```python
from build123d import *

# Parameters (mm, degrees)
SKETCH1_R         = 3.8608
EXTRUDE1_DEPTH    = 14.605
SKETCH2_OUTSIDE_W = 13.37
SKETCH2_OUTSIDE_H = 13.37
SKETCH2_OUTSIDE_R = 2.4892
EXTRUDE2_DEPTH    = 9.525
EXTRUDE3_DEPTH    = 3.048


with BuildPart() as part:
    # Sketch1 → Extrude1 (new body)
    with BuildSketch(Plane.XY):
        Circle(SKETCH1_R)
    extrude(amount=EXTRUDE1_DEPTH)

    # Sketch2 outside → Extrude2 (cut)
    with BuildSketch(Plane.XY.offset(14.605)):
        Rectangle(SKETCH2_OUTSIDE_W, SKETCH2_OUTSIDE_H)
        Circle(SKETCH2_OUTSIDE_R, mode=Mode.SUBTRACT)
    extrude(amount=-EXTRUDE2_DEPTH, mode=Mode.SUBTRACT)

    # Sketch3 → Extrude3 (cut)
    with BuildSketch(Plane(origin=(0, 0, 0), x_dir=(-1, 0, 0), z_dir=(0, 0, -1))):
        Polygon((0, 2.987683948), (-2.587410198, 1.493841974), (-2.587410198, -1.493841974), (0, -2.987683948), (2.587410198, -1.493841974), (2.587410198, 1.493841974), align=None)
    extrude(amount=-EXTRUDE3_DEPTH, mode=Mode.SUBTRACT)


solid = part.part
```
Model file for the job. Use its own axes, mm. A direction names the side the tool comes from. Give positions to 0.01 mm unless a question says otherwise; leave off trailing zeros. Loops run counter-clockwise (first coordinate to the right, second up) from the corner with the lowest first, then second, coordinate; pieces in that order, holes last. Notation, with made-up numbers: (-22, 4.5) -> (1, 4.5) arc R24 ccw to (1, 18.5) -> close; hole circle Ø5 at (-5, 71). An arc over 180 degrees is marked (long way). Write each question's results on one line, items separated by ' | '.
(1) Tool access for faces 1 (the flat face through (-1.31, 2.23, 1.5)), 2 (the flat face through (-3, 0, 0)), 3 (the cylindrical face through (2.374, 0.748, 9.909)): list every direction of +Z, -Z, +X, -X, +Y, -Y with a clear straight run to the whole face (end or side of a thin tool).
Geometry results:
face 1: -Z | face 2: -Z, +X, -X, +Y, -Y | face 3: +Z
(2) Probe line 1 along Z through (x, y) = (1.25, 1) (3 decimals); line 2 along Z through (x, y) = (-2.5, 2); line 3 along X through (y, z) = (0.5, 1.75). List the from-to ranges inside material, lowest first.
Geometry results:
line 1: z = 3.048 to 14.605 | line 2: z = 0 to 5.08 | line 3: x = -3.83 to -2.59, 2.59 to 3.83
(3) Cut at B-B on x = -2.25. List the corners of the cut face in (y, z) (3 decimals).
Geometry results:
outline: (-3.137, 0) -> (-1.689, 0) -> (-1.689, 3.048) -> (1.689, 3.048) -> (1.689, 0) -> (3.137, 0) -> (3.137, 5.08) -> (1.065, 5.08) -> (1.065, 14.605) -> (-1.065, 14.605) -> (-1.065, 5.08) -> (-3.137, 5.08) -> close
(4) Cut at C-C on z = 3.25. List the corners of the cut face in (x, y), and give its area (3 significant figures).
Geometry results:
outline: circle Ø7.72 at (0, 0) | area: 46.8 mm²
(5) Cut at D-D on z = 10.75. List the corners of the cut face in (x, y), and give its area (3 significant figures).
Geometry results:
outline: circle Ø4.98 at (0, 0) | area: 19.5 mm²
(6) Cut at A-A on y = 0. List the corners of the cut face in (x, z) (3 decimals), and give its area (3 significant figures).
Geometry results:
outline: (-3.861, 0) -> (-2.587, 0) -> (-2.587, 3.048) -> (2.587, 3.048) -> (2.587, 0) -> (3.861, 0) -> (3.861, 5.08) -> (2.489, 5.08) -> (2.489, 14.605) -> (-2.489, 14.605) -> (-2.489, 5.08) -> (-3.861, 5.08) -> close | area: 70.9 mm²
(7) Pull direction X, two halves, no side cores. Call faces 4 (the flat face through (3, 0, 5.08)), 5 (the cylindrical face through (-0.5, 3.83, 2.5)), 6 (the flat face through (-1.28, -2.25, 1.5)), 7 (the flat face through (2.587, 0, 2)): released by +X, released by -X, zero draft, split by the parting line, or undercut.
Geometry results:
face 4: zero draft | face 5: split by the parting line | face 6: undercut | face 7: undercut
(8) Flat gauge pins, fed straight in: pin 1 Ø1 at (x, z) = (-1, 7) entering from +Y; pin 2 Ø2.5 at (x, y) = (0, -1) entering from -Z; pin 3 Ø3 at (y, z) = (-2.5, 5.5) entering from -X. Where does each tip first touch, or does it go through?
Geometry results:
pin 1: stops at y = 2.44 | pin 2: stops at z = 3.05 | pin 3: stops at x = -3.71
